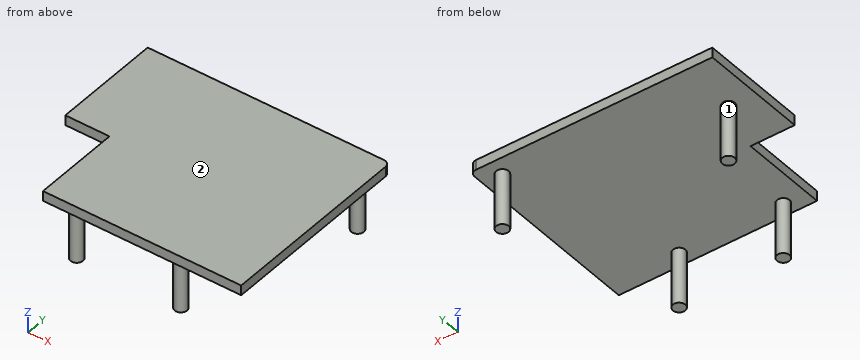
from build123d import *

# Parameters (mm, degrees)
BOSS_EXTRUDE1_DEPTH = 1.6
SKETCH5_R           = 1
BOSS_EXTRUDE2_DEPTH = 9


with BuildPart() as part:
    # Sketch4 → Boss-Extrude1 (new body)
    with BuildSketch(Plane.XY):
        with BuildLine():
            Line((214.083314686, -91.426205385), (214.083314686, -108.78795934))
            Line((214.083314686, -108.78795934), (221.166748687, -108.78795934))
            Line((221.166748687, -108.78795934), (221.166748687, -122.793871773))
            Line((221.166748687, -122.793871773), (252.95, -122.793871773))
            Line((252.95, -122.793871773), (252.95, -92.4019243))
            ThreePointArc((252.95, -92.4019243), (252.656880102, -91.694590841), (251.949358863, -91.401924489))
            Line((251.949358863, -91.401924489), (214.083314686, -91.426205385))
        make_face()
    extrude(amount=BOSS_EXTRUDE1_DEPTH)

    # Sketch5 → Boss-Extrude2 (add)
    with BuildSketch(Plane(origin=(0, 0, 0), x_dir=(-1, 0, 0), z_dir=(0, 0, -1))):
        with Locations((-224.853507667, -120.53205767)):
            Circle(SKETCH5_R)
        with Locations((-218.408459116, -100.527296583)):
            Circle(SKETCH5_R)
        with Locations((-241.552042549, -120.53205767)):
            Circle(SKETCH5_R)
        with Locations((-249.796682579, -94.124098997)):
            Circle(SKETCH5_R)
    extrude(amount=BOSS_EXTRUDE2_DEPTH)


solid = part.part
Source: CAD feature listing. Evaluate the final solid. Frame: model axes, mm. Face numbers are marked on the shaded views. A direction names the side the tool comes from. Round coordinates to 2 decimals unless told otherwise and drop trailing zeros. Order: outer loops, then holes, each group sorted by start corner. A loop starts at its lowest first (then second) coordinate and runs counter-clockwise, first axis right, second up. Notation, with made-up numbers: (87, 0) - (120, 0) arc R32 cw to (120, 34) - close; hole circle Ø1 at (40.5, 82.5). An arc over 180 degrees is marked (long way). Use a Markdown table: item, result. Add a question column.
1. Set-up query: the marked faces 1 and 2. Return all of +Z, -Z, +X, -X, +Y, -Y with unobstructed straight access to the full face (end or side cutting, diameter ignored); none if empty.
2. Section query A-A (z = -4.5). Return the cut outline in (x, y), then the cut area to 3 significant figures.
3. Section query D-D (y = -112). Return the cut outline in (x, z).
4. Section query B-B (y = -100). Return the cut outline in (x, z).
5. First-contact query: pin 1 (1.5 mm diameter, centred on y = -99.5, z = -5, fed in from +X); pin 2 (5 mm diameter, centred on x = 243.5, z = -7, fed in from -Y); pin 3 (3 mm diameter, centred on x = 240.5, y = -103, fed in from -Z). Flat tips, straight axial feed; report the tip coordinate or a pass-through.
6. Section query C-C (x = 225). Return the cut outline in (y, z), then the cut area to 3 significant figures.
7. Line query: probe 1 along Y at (x, z) = (246, 0.5); probe 2 along Z at (x, y) = (239, -107.5); probe 3 along Y at (x, z) = (225, -3.75). Output: solid intervals per line, ascending.
Derived:
| question | item | result |
|---|---|---|
| 1 | face 1 | -Z |
| 1 | face 2 | +Z, +X, -X, +Y, -Y |
| 2 | outline | circle Ø2 at (218.41, -100.53); circle Ø2 at (224.85, -120.53); circle Ø2 at (241.55, -120.53); circle Ø2 at (249.8, -94.12) |
| 2 | area | 12.6 mm2 |
| 3 | outline | (221.17, 0) - (252.95, 0) - (252.95, 1.6) - (221.17, 1.6) - close |
| 4 | outline | (214.08, 0) - (217.56, 0) - (217.56, -9) - (219.26, -9) - (219.26, 0) - (252.95, 0) - (252.95, 1.6) - (214.08, 1.6) - close |
| 5 | pin 1 | x = 219.37 |
| 5 | pin 2 | y = -121.53 |
| 5 | pin 3 | z = 0 |
| 6 | outline | (-122.79, 0) - (-121.52, 0) - (-121.52, -9) - (-119.54, -9) - (-119.54, 0) - (-91.42, 0) - (-91.42, 1.6) - (-122.79, 1.6) - close |
| 6 | area | 68.0 mm2 |
| 7 | probe 1 | -122.79 to -91.41 |
| 7 | probe 2 | 0 to 1.6 |
| 7 | probe 3 | -121.52 to -119.54 |
